Part model, mm, in its own coordinate system. A direction names the side the tool comes from. Coordinates: 2 decimals unless noted, no trailing zeros. Write each loop counter-clockwise with the first axis right and the second up, starting at its lowest first coordinate (ties: lowest second). Pieces come first, ordered by that corner, then holes. Notation, with made-up numbers: (-22.75, 69.25) - (9.25, 69.25) arc R12 ccw to (9.25, 81.25) - close; hole circle Ø2 at (-38.75, 69). An arc over 180 degrees is marked (long way). Use a Markdown table: item, result.
```python
from build123d import *

# Parameters (mm, degrees)
EXTRUDE_1_DEPTH     = 15
SKETCH_2_W          = 60
SKETCH_2_H          = 43
CUT_EXTRUDE_1_DEPTH = 1
EXTRUDE_START       = 46
SKETCH_3_W          = 142
SKETCH_3_H          = 98
EXTRUDE_2_DEPTH     = 1.5
EXTRUDE_3_REACH     = 141.173
SKETCH_4_W          = 8.580803558
SKETCH_4_H          = 6.129145399
SKETCH_4_H_2        = 6.742059939
SKETCH_4_W_2        = 9.806632637
SKETCH_4_H_3        = 5.698922344
CHAMFER_1_SIZE      = 2
FILLET_1_R          = 2
SKETCH_5_W          = 58.826750964
SKETCH_5_H          = 40.858747532
EXTRUDE_4_DEPTH     = 19
SKETCH_6_W          = 82.94818023
SKETCH_6_H          = 52.919462164
EXTRUDE_5_DEPTH     = 10


with BuildPart() as part:
    # Sketch 1 → Extrude 1 (new body)
    with BuildSketch(Plane(origin=(0, 0, 0), x_dir=(1, 0, 0), z_dir=(0, 1, 0))):
        with BuildLine():
            Line((61, 68.869441699), (61, 25))
            Line((61, 25), (88.53812738, 25))
            ThreePointArc((88.53812738, 25), (0, -92), (-88.53812738, 25))
            Line((-88.53812738, 25), (-61, 25))
            Line((-61, 25), (-61, 68.869441699))
            ThreePointArc((-61, 68.869441699), (0, 92), (61, 68.869441699))
        make_face()
    extrude(amount=EXTRUDE_1_DEPTH)

    # Sketch 2 → Cut-Extrude 1 (cut)
    with BuildSketch(Plane.XZ):
        with Locations((0, 71.283217175)):
            Rectangle(SKETCH_2_W, SKETCH_2_H)
    extrude(amount=-CUT_EXTRUDE_1_DEPTH, mode=Mode.SUBTRACT)


with BuildPart() as body_2:
    # Sketch 3 → Extrude 2 (new body)
    with BuildSketch(Plane(origin=(0, 15, 0), x_dir=(1, 0, 0), z_dir=(0, 1, 0)).offset(EXTRUDE_START)):
        with Locations((-22, -2)):
            Rectangle(SKETCH_3_W, SKETCH_3_H)
    extrude(amount=EXTRUDE_2_DEPTH)

    # Sketch 4 → Extrude 3 (add, up to next)
    with BuildSketch(Plane(origin=(0, 15, 0), x_dir=(1, 0, 0), z_dir=(0, 1, 0)), mode=Mode.PRIVATE) as extrude_3_sk1:
        with Locations((39.89053511, 37.643718522)):
            Rectangle(SKETCH_4_W, SKETCH_4_H)
    extrude_3_tool1 = extrude(extrude_3_sk1.sketch, amount=EXTRUDE_3_REACH, mode=Mode.PRIVATE) - body_2.part
    # Sketch 4 → Extrude 3 (add, up to next)
    with BuildSketch(Plane(origin=(0, 15, 0), x_dir=(1, 0, 0), z_dir=(0, 1, 0)), mode=Mode.PRIVATE) as extrude_3_sk2:
        with Locations((39.89053511, -40.502885308)):
            Rectangle(SKETCH_4_W, SKETCH_4_H_2)
    extrude_3_tool2 = extrude(extrude_3_sk2.sketch, amount=EXTRUDE_3_REACH, mode=Mode.PRIVATE) - body_2.part
    # Sketch 4 → Extrude 3 (add, up to next)
    with BuildSketch(Plane(origin=(0, 15, 0), x_dir=(1, 0, 0), z_dir=(0, 1, 0)), mode=Mode.PRIVATE) as extrude_3_sk3:
        with Locations((-70.127624791, -40.502885308)):
            Rectangle(SKETCH_4_W_2, SKETCH_4_H_2)
    extrude_3_tool3 = extrude(extrude_3_sk3.sketch, amount=EXTRUDE_3_REACH, mode=Mode.PRIVATE) - body_2.part
    # Sketch 4 → Extrude 3 (add, up to next)
    with BuildSketch(Plane(origin=(0, 15, 0), x_dir=(1, 0, 0), z_dir=(0, 1, 0)), mode=Mode.PRIVATE) as extrude_3_sk4:
        with Locations((-70.127624791, 18.84767654)):
            Rectangle(SKETCH_4_W_2, SKETCH_4_H_3)
    extrude_3_tool4 = extrude(extrude_3_sk4.sketch, amount=EXTRUDE_3_REACH, mode=Mode.PRIVATE) - body_2.part

    add(part.part)  # Extrude 3 merges part
    add(extrude_3_tool1.solids().sort_by_distance((39.890535, 15, -37.643719))[0])
    add(extrude_3_tool2.solids().sort_by_distance((39.890535, 15, 40.502885))[0])
    add(extrude_3_tool3.solids().sort_by_distance((-70.127625, 15, 40.502885))[0])
    add(extrude_3_tool4.solids().sort_by_distance((-70.127625, 15, -18.847677))[0])

    # Chamfer 1
    chamfer_1_edges = [body_2.edges().sort_by_distance(p)[0] for p in [
        (0, 15, 92),
    ]]
    chamfer(chamfer_1_edges, length=CHAMFER_1_SIZE)

    # Fillet 1
    fillet_1_edges = [body_2.edges().sort_by_distance(p)[0] for p in [
        (0, 15, -92),
    ]]
    fillet(fillet_1_edges, radius=FILLET_1_R)

    # Sketch 5 → Extrude 4 (add)
    with BuildSketch(Plane.XZ):
        with Locations((-46.404556715, 7.01490545)):
            Rectangle(SKETCH_5_W, SKETCH_5_H)
    extrude(amount=EXTRUDE_4_DEPTH)

    # Sketch 6 → Extrude 5 (add)
    with BuildSketch(Plane(origin=(0, 15, 0), x_dir=(1, 0, 0), z_dir=(0, 1, 0))):
        with Locations((43.681597482, -9.107070233)):
            Rectangle(SKETCH_6_W, SKETCH_6_H)
    extrude(amount=EXTRUDE_5_DEPTH)


solid = body_2.part
```
Item 1: Band-saw the part on B-B, the plane y = 33.5. Give the cut face in (x, z), then the cut area to 3 significant figures.
From the geometry:
| item | result |
|---|---|
| outline | (-75.03, -21.7) - (-65.22, -21.7) - (-65.22, -16) - (-75.03, -16) - close; (-75.03, 37.13) - (-65.22, 37.13) - (-65.22, 43.87) - (-75.03, 43.87) - close; (35.6, -40.71) - (44.18, -40.71) - (44.18, -34.58) - (35.6, -34.58) - close; (35.6, 37.13) - (44.18, 37.13) - (44.18, 43.87) - (35.6, 43.87) - close |
| area | 232 mm^2 |
Item 2: Band-saw the part on A-A, the plane z = 0. Give the cut face in (x, y).
From the geometry:
| item | result |
|---|---|
| outline | (-93, 61) - (49, 61) - (49, 62.5) - (-93, 62.5) - close; (-92, 0) - (-75.82, 0) - (-75.82, -19) - (-16.99, -19) - (-16.99, 0) - (92, 0) - (92, 13) - (90, 15) - (85.16, 15) - (85.16, 25) - (2.21, 25) - (2.21, 15) - (-90, 15) - (-92, 13) - close |
Item 3: Which spindle directions (+Z, -Z, +X, -X, +Y, -Y) get a long thin tool onto all of the face, cutting with end or side? Do faces 1 (the face through (-75, 7, -25)), 2 (the face through (2.38, 6.41, 91.97)), 3 (the face through (44.181, 38, 41)). Say none if no direction does.
From the geometry:
| item | result |
|---|---|
| face 1 | -Z, -X, -Y |
| face 2 | -Y |
| face 3 | +Z, +X |
Item 4: Drop flat-ended pins along their axis: P1, Ø11, axis at x = 50.5, y = 21, coming from the -Z side; P2, Ø11, axis at x = -69.5, y = 48.5, coming from the -Z side; P3, Ø1.7, axis at y = 40.5, z = -18.5, coming from the +X side. Give the stop position or say it passes through.
From the geometry:
| item | result |
|---|---|
| P1 | z = -17.35 |
| P2 | z = -21.7 |
| P3 | x = -65.22 |
Item 5: Drill centre lines: probe 1 along Y at (x, z) = (1, 47); probe 2 along X at (y, z) = (39.5, 38.5); probe 3 along Y at (x, z) = (-66, -12). Where is each one in solid material? Low to high.
From the geometry:
| item | result |
|---|---|
| probe 1 | 0 to 15, 61 to 62.5 |
| probe 2 | -75.03 to -65.22, 35.6 to 44.18 |
| probe 3 | -19 to 15, 61 to 62.5 |
Item 6: Two-plate mould, pull along Y, no slides. Class faces 4 (the face through (-47, -9, -13.414)), 5 (the face through (-75.031, 38, -19)), 6 (the face through (-47, -19, 7)): pulls with the +Y half, pulls with the -Y half, needs draft (parallel to the pull), parting line crosses it, or undercut.
From the geometry:
| item | result |
|---|---|
| face 4 | needs draft |
| face 5 | undercut |
| face 6 | pulls with the -Y half |
Item 7: Band-saw the part on C-C, the plane x = 0. Give the cut face in (y, z), then the cut area to 3 significant figures.
From the geometry:
| item | result |
|---|---|
| outline | (0, -92) - (13, -92) arc R2 ccw to (15, -90) - (15, 90) - (13, 92) - (1, 92) - (1, 49.78) - (0, 49.78) - close; (61, -47) - (62.5, -47) - (62.5, 51) - (61, 51) - close |
| area | 2,860 mm^2 |
Item 8: Band-saw the part on D-D, the plane y = 6. Give the cut face in (x, z), then the cut area to 3 significant figures.
From the geometry:
| item | result |
|---|---|
| outline | (-88.54, -25) - (-61, -25) - (-61, -68.87) arc R92 ccw to (61, -68.87) - (61, -25) - (88.54, -25) arc R92 ccw (long way) to start |
| area | 25,100 mm^2 |
